Autodesk Inventor part; units mm, degrees
ref_plane "YZ Plane" through (0, 0, 0) normal (1, 0, 0) x (0, 1, 0)
ref_plane "XZ Plane" through (0, 0, 0) normal (0, 1, 0) x (-1, 0, 0)
ref_plane "XY Plane" through (0, 0, 0) normal (0, 0, 1) x (1, 0, 0)
sketch "Sketch1" plane through (0, 0, 0) normal (1, 0, 0) x (0, 1, 0)
  point P0 (0, 0)
sketch "Sketch2" plane through (0, 0, 0) normal (0, 1, 0) x (-1, 0, 0)
  point P0 (0, 0)
sketch "Sketch3" plane through (0, 0, 0) normal (0, 1, 0) x (-1, 0, 0)
  line L0 (0, 0) -> (-15, 0)
  line L1 (-15, 0) -> (-15, -35)
  line L2 (-15, -35) -> (0, -35)
  line L3 (0, -35) -> (0, 0)
  dimension "d0" = 35
  dimension "d1" = 15
extrude "Extrusion1" add sketch "Sketch3" along normal blind 3.5
sketch "Sketch4" plane through (0, 0, 0) normal (0, -1, 0) x (1, 0, 0)
  point P0 (0, 0)
sketch "Sketch5" plane through (0, 0, 0) normal (0, -1, 0) x (1, 0, 0)
  line L0 (15, 0) -> (15, -35)
  line L1 (15, 0) -> (0, 0)
  line L2 (0, 0) -> (0, -6.5)
  line L3 (0, -6.5) -> (15, -6.5)
  line L4 (15, -6.5) -> (15, 0)
  line L5 (0, -35) -> (0, 0)
  line L6 (15, -35) -> (0, -35)
  line L7 (0, -35) -> (0, -28.5)
  line L8 (0, -28.5) -> (15, -28.5)
  line L9 (15, -28.5) -> (15, -35)
  dimension "d4" = 6.5
  dimension "d5" = 6.5
extrude "Extrusion2" add sketch "Sketch5" along normal blind 12 contours L0 L3 L2 L1 | L0 L6 L5 L8
fillet "Fillet2" radius 3.5875 2 edges at (7.5, 3.5, -35) (7.5, 3.5, 0)
sketch "Sketch7" plane through (0, 3.5, 0) normal (0, 1, 0) x (1, 0, 0)
  point P0 (0, 0)
sketch "Sketch8" plane through (0, -12, 0) normal (0, -1, 0) x (1, 0, 0)
  circle A0 centre (7.5, 7) radius 7
  circle A1 centre (7.5, -42) radius 7
  line L0 (15, 0) -> (0, 0)
  line L1 (0, -35) -> (15, -35)
  circle A2 centre (7.5, 7) radius 3.5
  circle A3 centre (7.5, -42) radius 3.5
  line L2 (0, 0) -> (15, 0)
  line L3 (13.5622, 0) -> (1.4378, 0)
  line L4 (1.4378, 0) -> (1.4378, 3.5)
  line L5 (1.4378, 3.5) -> (13.5622, 3.5)
  line L6 (13.5622, 3.5) -> (13.5622, 0)
  line L7 (13.5622, -35) -> (1.4378, -35)
  line L8 (1.4378, -35) -> (1.4378, -38.5)
  line L9 (1.4378, -38.5) -> (13.5622, -38.5)
  line L10 (13.5622, -38.5) -> (13.5622, -35)
  point P0 (7.5, 0)
  point P1 (7.5, -35)
  dimension "d14" = 14
  dimension "d15" = 14
  dimension "d16" = 7
  dimension "d17" = 7
extrude "Extrusion4" add sketch "Sketch8" against normal blind 12 contours A0 L5 | L5 A0 | L6 L0 A0 | A1 L9 | L9 A1 | A1 L1 L10 | L8 L1 A1
sketch "Sketch9" plane through (0, -12, 0) normal (0, -1, 0) x (1, 0, 0)
  line L0 (7.5, 0) -> (13.5622, 0)
  line L1 (7.5, 0) -> (1.4378, 0)
  line L2 (1.4378, 0) -> (1.4378, 3.5)
  line L3 (1.4378, 3.5) -> (7.5, 3.5)
  line L4 (7.5, 3.5) -> (7.5, 0)
  arc A0 (13.5622, 3.5) -> (7.5, 0) centre (7.5, 7) ccw
  point P0 (0, 0)
extrude "Extrusion5" add sketch "Sketch9" against normal blind 12
sketch "Sketch10" plane through (0, -12, 0) normal (0, -1, 0) x (1, 0, 0)
  line L0 (15, 0) -> (13.5622, 0)
  line L1 (15, 0) -> (0, 0)
  line L2 (0, 0) -> (0, 14.6227)
  line L3 (0, 14.6227) -> (15, 14.6227)
  line L4 (15, 14.6227) -> (15, 0)
  line L5 (15, -31.4125) -> (15, -35)
  line L6 (15, -35) -> (0, -35)
  line L7 (0, -35) -> (0, -49.9262)
  line L8 (0, -49.9262) -> (15, -49.9262)
  line L9 (15, -49.9262) -> (15, -35)
  point P0 (0, 0)
extrude "Extrusion6" cut sketch "Sketch10" against normal blind 2
sketch "Sketch11" plane through (0, -12, 0) normal (0, -1, 0) x (1, 0, 0)
  line L0 (0, -6.5) -> (15, -6.5)
  line L1 (0, -6.5) -> (15, -6.5)
  line L2 (15, -6.5) -> (15, -7.7)
  line L3 (15, -7.7) -> (0, -7.7)
  line L4 (0, -7.7) -> (0, -6.5)
  line L5 (15, -6.5) -> (15, -28.5)
  line L6 (0, -28.5) -> (0, -6.5)
  line L7 (15, -28.5) -> (0, -28.5)
  line L8 (0, -28.5) -> (0, -27.3)
  line L9 (0, -27.3) -> (15, -27.3)
  line L10 (15, -27.3) -> (15, -28.5)
  point P0 (0, 0)
  dimension "d24" = 1.2
  dimension "d25" = 1.2
extrude "Extrusion7" add sketch "Sketch11" against normal blind 12 contours L0 L2 L3 L4 | L9 L5 L7 L6
fillet "Fillet4" radius 2 2 edges at (7.5, 0, -7.7) (7.5, 0, -27.3)
properties part number "HP45 Printhead Cap"
Could you check a few things on this model? Use its own coordinates, in mm. A direction names the side the tool comes from. Coordinates: 2 decimals unless noted, no trailing zeros. Loops run counter-clockwise (first coordinate to the right, second up) from the corner with the lowest first, then second, coordinate; pieces in that order, holes last. Notation, with made-up numbers: M 62,75 L 82,75 A15 cw 82,87 Z; hole C -35,-29.5 d9. An arc over 180 degrees is marked long. Put each result on its own line as item: value. Start each with the question number.
(1) For faces 1 (the face through (8, 0, -17)), 2 (the face through (4, -10, 9)), 3 (the face through (13.562, -5, -37)), 4 (the face through (4, -10, -40)), which set-ups out of +Z, -Z, +X, -X, +Y, -Y let a thin tool reach every point of the face, with its end or its side?
(2) Suppose I cut it at C-C on x = 7.5. Count the separate pieces of the cut face and the enclosed holes in it, then the cut area to 3 significant figures.
(3) Suppose I cut it at D-D on z = -23.5. Please give me the cut outline in (x, y), then the cut area to 3 significant figures.
(4) Thinking about a two-plate mould opening in Z: for faces 5 (the face through (4, 0, -40)), 6 (the face through (8, -11, -35)), which applies, pulls with the +Z half, pulls with the -Z half, needs draft (parallel to the pull), parting line crosses it, or undercut?
(5) Will these pins go through, and if not, where does the flat tip stop? P1, Ø1.8, axis at y = -3.5, z = -36.5, coming from the -X side; P2, Ø1, axis at y = -4.5, z = -36.5, coming from the +X side; P3, Ø2, axis at x = 2, y = 0.5, coming from the -Z side.
(6) Suppose I cut it at B-B on y = -3.25. Please give me the cut outline in (x, z).
(7) I need wall thicknesses on line 1 (X direction, y = -2.25, z = 7); line 2 (Y direction, x = 8.5, z = 3.5); line 3 (Z direction, x = 9, y = -7). Which ranges of each line are inside material? Lowest first, please. Write a range as from..to.
(8) Suppose I cut it at A-A on z = 7. Please give me the cut outline in (x, y), then the cut area to 3 significant figures.
Solutions:
1. face 1: +X, -X, -Y
1. face 2: +Z, +X, -X, -Y
1. face 3: +X, +Y, -Y
1. face 4: -Z, +X, -X, -Y
2. separate pieces: 3
2. enclosed holes: 0
2. area: 443 mm2
3. outline: M 0,0 L 15,0 L 15,3.5 L 0,3.5 Z
3. area: 52.5 mm2
4. face 5: needs draft
4. face 6: undercut
5. P1: stops at x = 1.44
5. P2: stops at x = 13.56
5. P3: stops at z = -47.25
6. outline: M 0,-35 L 1.44,-35 L 1.44,-38.5 A7 ccw long 13.56,-38.5 L 13.56,-35 L 15,-35 L 15,-27.3 L 0,-27.3 Z; M 0,-7.7 L 15,-7.7 L 15,0 L 13.56,0 L 13.56,3.5 A7 ccw long 1.44,3.5 L 1.44,0 L 0,0 Z; hole C 7.5,-42 d7; hole C 7.5,7 d7
7. line 1: x = 0.5..4, 11..14.5
7. line 2: y = -10..0
7. line 3: z = -48.84..-45.16, -38.84..-27.3, -7.7..3.84, 10.16..13.84
8. outline: M 0.5,-10 L 4,-10 L 4,0 L 0.5,0 Z; M 11,-10 L 14.5,-10 L 14.5,0 L 11,0 Z
8. area: 70.0 mm2
